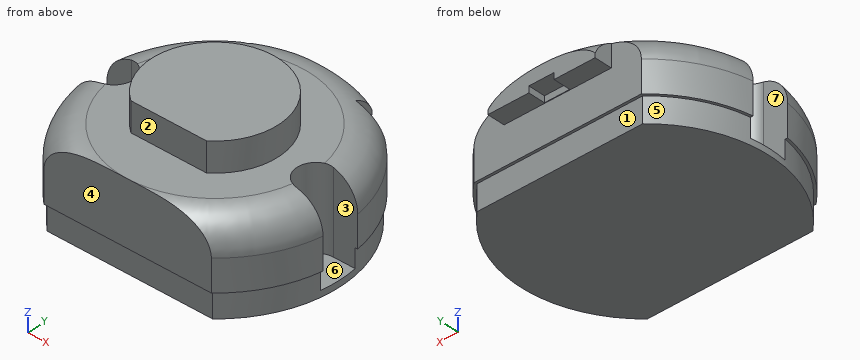
```python
from build123d import *

# Parameters (mm, degrees)
BOX010_W          = 30
BOX010_H          = 10
BOX010_DEPTH      = 30
BOX011_W          = 30
BOX011_H          = 10
BOX011_DEPTH      = 30
CYLINDER003_R     = 10.05
CYLINDER003_DEPTH = 20
FILLET002_R       = 2
THICKNESS_T       = -0.2
BOX017_W          = 20
BOX017_H          = 10
BOX017_DEPTH      = 10
CYLINDER005_R     = 5
CYLINDER005_DEPTH = 3.3
PAD002_DEPTH      = 20
BOX016_W          = 2
BOX016_H          = 2
BOX016_DEPTH      = 2
BOX015_W          = 30
BOX015_H          = 10
BOX015_DEPTH      = 30
BOX013_W          = 30
BOX013_H          = 10
BOX013_DEPTH      = 30
BOX014_W          = 8.5
BOX014_H          = 2.4
BOX014_DEPTH      = 44
BOX012_W          = 30
BOX012_H          = 10
BOX012_DEPTH      = 30
CYLINDER004_R     = 10.05
CYLINDER004_DEPTH = 7
FILLET003_R       = 2.5


with BuildPart() as cubo011:
    # Box010 → Box010 (new body)
    with BuildSketch(Plane(origin=(-15, 7.55, -3), x_dir=(1, 0, 0), z_dir=(0, 0, 1))):
        with Locations((15, 5)):
            Rectangle(BOX010_W, BOX010_H)
    extrude(amount=BOX010_DEPTH)


with BuildPart() as cubo012:
    # Box011 → Box011 (new body)
    with BuildSketch(Plane(origin=(-15, -17.55, -3), x_dir=(1, 0, 0), z_dir=(0, 0, 1))):
        with Locations((15, 5)):
            Rectangle(BOX011_W, BOX011_H)
    extrude(amount=BOX011_DEPTH)


with BuildPart() as thickness:
    # Cylinder003 → Cylinder003 (new body)
    with BuildSketch(Plane.XY):
        Circle(CYLINDER003_R)
    extrude(amount=CYLINDER003_DEPTH)

    # Fillet002
    fillet002_edges = [thickness.edges().sort_by_distance(p)[0] for p in [
        (-10.05, 0, 0),
    ]]
    fillet(fillet002_edges, radius=FILLET002_R)

    # Cut010: cut Cubo012
    add(cubo012.part, mode=Mode.SUBTRACT)

    # Cut011: cut Cubo011
    add(cubo011.part, mode=Mode.SUBTRACT)

    # Thickness
    thickness_openings = [thickness.faces().sort_by_distance(p)[0] for p in [
        (0, 0, 20),
    ]]
    offset(amount=THICKNESS_T, openings=thickness_openings)


with BuildPart() as cubo018:
    # Box017 → Box017 (new body)
    with BuildSketch(Plane(origin=(-10, -14, -3), x_dir=(1, 0, 0), z_dir=(0, 0, 1))):
        with Locations((10, 5)):
            Rectangle(BOX017_W, BOX017_H)
    extrude(amount=BOX017_DEPTH)


with BuildPart() as obj1:
    # Cylinder005 → Cylinder005 (new body)
    with BuildSketch(Plane.XY):
        Circle(CYLINDER005_R)
    extrude(amount=CYLINDER005_DEPTH)

    # Cut017: cut Cubo018
    add(cubo018.part, mode=Mode.SUBTRACT)


with BuildPart() as obj1_1:
    # Cut017 placement: moved
    add(obj1.part.moved(Location((0, 0, 6))))


with BuildPart() as pad002:
    # Sketch002 → Pad002 (new body)
    with BuildSketch(Plane.XY):
        with BuildLine():
            ThreePointArc((-10, 1.5), (-11.5, 0), (-10, -1.5))
            Line((-10, -1.5), (10, -1.5))
            ThreePointArc((10, -1.5), (11.5, 0), (10, 1.5))
            Line((-10, 1.5), (10, 1.5))
        make_face()
    extrude(amount=PAD002_DEPTH)


with BuildPart() as clone_of_pad004:
    # Clone004 base: copy of Pad002
    add(pad002.part)


with BuildPart() as clone_of_pad004_1:
    # Clone004 placement: moved
    add(clone_of_pad004.part.moved(Location((18, 0, 0.5))))


with BuildPart() as clone_of_pad003:
    # Clone003 base: copy of Pad002
    add(pad002.part)


with BuildPart() as clone_of_pad003_1:
    # Clone003 placement: moved
    add(clone_of_pad003.part.moved(Location((-18, 0, 0.5))))


with BuildPart() as cubo017:
    # Box016 → Box016 (new body)
    with BuildSketch(Plane(origin=(-1, 7.6, 3.5), x_dir=(1, 0, 0), z_dir=(0, 0, 1))):
        with Locations((1, 1)):
            Rectangle(BOX016_W, BOX016_H)
    extrude(amount=BOX016_DEPTH)


with BuildPart() as cubo016:
    # Box015 → Box015 (new body)
    with BuildSketch(Plane(origin=(-15, 7.55, -25), x_dir=(1, 0, 0), z_dir=(0, 0, 1))):
        with Locations((15, 5)):
            Rectangle(BOX015_W, BOX015_H)
    extrude(amount=BOX015_DEPTH)


with BuildPart() as cubo014:
    # Box013 → Box013 (new body)
    with BuildSketch(Plane(origin=(-15, -17.55, -3), x_dir=(1, 0, 0), z_dir=(0, 0, 1))):
        with Locations((15, 5)):
            Rectangle(BOX013_W, BOX013_H)
    extrude(amount=BOX013_DEPTH)


with BuildPart() as cubo015:
    # Box014 → Box014 (new body)
    with BuildSketch(Plane(origin=(-4.25, 6.55, -4), x_dir=(1, 0, 0), z_dir=(0, 0, 1))):
        with Locations((4.25, 1.2)):
            Rectangle(BOX014_W, BOX014_H)
    extrude(amount=BOX014_DEPTH)


with BuildPart() as cut012:
    # Box012 → Box012 (new body)
    with BuildSketch(Plane(origin=(-15, 7.55, -3), x_dir=(1, 0, 0), z_dir=(0, 0, 1))):
        with Locations((15, 5)):
            Rectangle(BOX012_W, BOX012_H)
    extrude(amount=BOX012_DEPTH)

    # Cut012: cut Cubo015
    add(cubo015.part, mode=Mode.SUBTRACT)


with BuildPart() as cut012_1:
    # Cut012 placement: moved
    add(cut012.part.moved(Location((0, 0, -12))))


with BuildPart() as tapa:
    # Cylinder004 → Cylinder004 (new body)
    with BuildSketch(Plane.XY):
        Circle(CYLINDER004_R)
    extrude(amount=CYLINDER004_DEPTH)

    # Fillet003
    fillet003_edges = [tapa.edges().sort_by_distance(p)[0] for p in [
        (-10.05, 0, 7),
    ]]
    fillet(fillet003_edges, radius=FILLET003_R)

    # Cut013: cut Cut012
    add(cut012_1.part, mode=Mode.SUBTRACT)

    # Cut014: cut Cubo014
    add(cubo014.part, mode=Mode.SUBTRACT)

    # Cut015: cut Cubo016
    add(cubo016.part, mode=Mode.SUBTRACT)

    # Cut016: cut Cubo017
    add(cubo017.part, mode=Mode.SUBTRACT)

    # Cut018: cut Clone of Pad003
    add(clone_of_pad003_1.part, mode=Mode.SUBTRACT)

    # Cut019: cut Clone of Pad004
    add(clone_of_pad004_1.part, mode=Mode.SUBTRACT)

    # Fusion002: union obj1
    add(obj1_1.part)


with BuildPart() as tapa_1:
    # Fusion002 placement: moved
    add(tapa.part.moved(Location((0, 0, 18))))

    # Cut020: cut Thickness
    add(thickness.part, mode=Mode.SUBTRACT)


solid = tapa_1.part
```
Build history of the part. All positions in model axes, mm. Face numbers are marked on the shaded views. A direction names the side the tool comes from. Round coordinates to 2 decimals unless told otherwise and drop trailing zeros. Loops run counter-clockwise (first coordinate to the right, second up) from the corner with the lowest first, then second, coordinate; pieces in that order, holes last.
Item 1: Saw through at B-B (z = 21). List the corners of the cut face in (x, y).
Item 2: Saw through at A-A (y = 0). List the corners of the cut face in (x, z).
Item 3: Which spindle directions (+Z, -Z, +X, -X, +Y, -Y) get a long thin tool onto all of the face, cutting with end or side? Do the marked faces 1, 2 and 3. Say none if no direction does.
Item 4: Pin check, flat tips, straight feed: P1, Ø2, axis at x = 3.5, z = 25.5, coming from the +Y side; P2, Ø0.7, axis at y = 8.5, z = 23.5, coming from the +X side; P3, Ø0.6, axis at x = 8.5, z = 22, coming from the +Y side. Stop position of each tip, or through.
Item 5: Drill centre lines: line 1 along X through (y, z) = (0, 21); line 2 along Z through (x, y) = (6, 3.5); line 3 along Y through (x, z) = (1.5, 20.25). Where is each one in solid material? Low to high.
Item 6: Two-plate mould, pull along Y, no slides. Class the marked faces 4, 5, 6 and 7: released by +Y, released by -Y, zero draft, split by the parting line, or undercut.
Item 7: Saw through at C-C (z = 26). List the corners of the cut face in (x, y).
Worked answers:
1. outline: (-9.94, -1.5) arc R10.05 ccw to (-6.63, -7.55) - (6.63, -7.55) arc R10.05 ccw to (9.94, -1.5) - (8, -1.5) arc R1.5 cw to (8, 1.5) - (9.94, 1.5) arc R10.05 ccw to (6.63, 7.55) - (-6.63, 7.55) arc R10.05 ccw to (-9.94, 1.5) - (-8, 1.5) arc R1.5 cw to (-8, -1.5) - close
2. outline: (-9.85, 18) - (9.85, 18) - (9.85, 18.5) - (6.5, 18.5) - (6.5, 25) - (5, 25) - (5, 27.3) - (-5, 27.3) - (-5, 25) - (-6.5, 25) - (-6.5, 18.5) - (-9.85, 18.5) - close
3. face 1: -Z, +X, -X, +Y
3. face 2: +Z, +X, -X, -Y
3. face 3: +Z, +X
4. P1: stops at y = 8.4
4. P2: stops at x = 4.25
4. P3: stops at y = 5.81
5. line 1: x = -6.5 to 6.5
5. line 2: z = 18 to 25
5. line 3: y = -7.55 to 7.55
6. face 4: released by -Y
6. face 5: split by the parting line
6. face 6: undercut
6. face 7: undercut
7. outline: (-3, -4) - (3, -4) arc R5 ccw (long way) to start
